The model under review builds one solid part; all positions refer to its coordinate system, in mm. Coordinates: 2 decimals unless noted, no trailing zeros. Loops run counter-clockwise (first coordinate to the right, second up) from the corner with the lowest first, then second, coordinate; pieces in that order, holes last. Notation, with made-up numbers: M 34.25,41.5 L 71.25,41.5 A6 cw 71.25,48.5 Z; hole C -29.5,-17 d4. An arc over 180 degrees is marked long. One line per item, written item: value.
Autodesk Inventor part; units mm, degrees
ref_plane "YZ Plane" through (0, 0, 0) normal (1, 0, 0) x (0, 1, 0)
ref_plane "XZ Plane" through (0, 0, 0) normal (0, 1, 0) x (-1, 0, 0)
ref_plane "XY Plane" through (0, 0, 0) normal (0, 0, 1) x (1, 0, 0)
sketch "Sketch2" plane through (0, 0, 0) normal (0, 1, 0) x (-1, 0, 0)
  line L0 (0, 0) -> (109, 0)
  line L1 (109, 0) -> (109, -44)
  line L2 (109, -44) -> (0, -44)
  line L3 (0, -44) -> (0, 0)
  line L4 (44, 0) -> (44, -44) construction
  arc A0 (87, -44) -> (87, 0) centre (87, -22) ccw
  circle A1 centre (94, -22) radius 5.1
  circle A2 centre (29.3333, -14.6667) radius 1.675
  circle A3 centre (29.3333, -29.3333) radius 1.675
  circle A4 centre (14.6667, -11) radius 1.675
  circle A5 centre (14.6667, -22) radius 1.675
  circle A6 centre (14.6667, -33) radius 1.675
  dimension "d36" = 44
  dimension "d37" = 44
  dimension "d38" = 65
  dimension "d41" = 10.2
  dimension "d42" = 22
  dimension "d43" = 15
  dimension "d44" = 14.6667
  dimension "d45" = 14.6667
  dimension "d46" = 14.6667
  dimension "d47" = 11
  dimension "d48" = 11
  dimension "d49" = 11
  dimension "d50" = 11
  dimension "d51" = 3.35
  dimension "d52" = 3.35
  dimension "d53" = 3.35
  dimension "d54" = 3.35
  dimension "d55" = 3.35
  dimension "d56" = 14.6667
  dimension "d57" = 14.6667
  dimension "d58" = 14.6667
  dimension "d59" = 14.6667
extrude "Plate3" add sketch "Sketch2" along normal blind 2 contours L0 A0 L2 L3
equation "\"d42\" = 0.5 * d37"
equation "\"d44\" = 0.333333 * d37"
equation "\"d45\" = d44"
equation "\"d47\" = 0.25 * d37"
equation "\"d48\" = d47"
equation "\"d49\" = d47"
equation "\"d52\" = d51"
equation "\"d53\" = d51"
equation "\"d54\" = d51"
equation "\"d55\" = d51"
equation "\"d56\" = 0.333333 * d36"
equation "\"d57\" = d56"
equation "\"d58\" = d46"
equation "\"d59\" = d46"
equation "\"d60\" = Thickness"
equation "\"BendRadius\" = Thickness"
equation "\"BendReliefWidth\" = Thickness"
equation "\"BendReliefDepth\" = 0.5 * Thickness"
equation "\"CornerReliefSize\" = 4 * Thickness"
equation "\"MinimumRemnant\" = 2 * Thickness"
equation "\"TransitionRadius\" = BendRadius"
equation "\"JacobiRadiusSize\" = BendRadius"
equation "\"GapSize\" = Thickness"
properties part number "Beslag ekstra håndtag"
(1) Add section A-A on z = -22. State the section outline as (x, y) points.
Checks:
outline: M -109,0 L -99.1,0 L -99.1,2 L -109,2 Z; M -88.9,0 L -16.34,0 L -16.34,2 L -88.9,2 Z; M -12.99,0 L 0,0 L 0,2 L -12.99,2 Z
(2) Insertion check: pin 1 Ø3 at (x, z) = (-14.67, -11) entering from +Y; pin 2 Ø1 at (y, z) = (0.5, -18) entering from -X. Each pin has a flat end and moves straight along its axis. Give the tip position at first contact, or say it passes through.
Checks:
pin 1: through
pin 2: x = -108.72
(3) Add section C-C on y = 0.7. State the section outline as (x, z) points (3 decimals).
Checks:
outline: M -87,-44 L 0,-44 L 0,0 L -87,0 A22 ccw Z; hole C -94,-22 d10.2; hole C -29.333,-29.333 d3.35; hole C -29.333,-14.667 d3.35; hole C -14.667,-33 d3.35; hole C -14.667,-22 d3.35; hole C -14.667,-11 d3.35
(4) Draft analysis for pull direction Z (two halves, no side actions). For faces 1 (the face through (-109, 1, -22)), 2 (the face through (0, 1, -22)), 3 (the face through (-27.66, 0.99, -14.74)), state which applies: pulls with the +Z half, pulls with the -Z half, needs draft (parallel to the pull), parting line crosses it, or undercut.
Checks:
face 1: parting line crosses it
face 2: needs draft
face 3: undercut
(5) To check wall thickness, follow L1, parallel to Z at x = -94, y = 1.2; L2, parallel to X at y = 0.4, z = -21; L3, parallel to X at y = 1.15, z = -26. State the ranges of each line that lie inside material, in increasing order. Write a range as [from, to].
Checks:
L1: [-42.86, -27.1], [-16.9, -1.14]
L2: [-108.98, -99], [-89, -16.01], [-13.32, 0]
L3: [-108.63, -97.16], [-90.84, 0]
(6) Add section B-B on x = -94. State the section outline as (y, z) points, then the cut area to 3 significant figures.
Checks:
outline: M 0,-42.86 L 2,-42.86 L 2,-27.1 L 0,-27.1 Z; M 0,-16.9 L 2,-16.9 L 2,-1.14 L 0,-1.14 Z
area: 63.0 mm^2
